The listing builds one solid part. Answer for the finished solid, in the listing's coordinates (mm). Face numbers are marked on the shaded views. A direction names the side the tool comes from. Coordinates: 2 decimals unless noted, no trailing zeros. Loops run counter-clockwise (first coordinate to the right, second up) from the corner with the lowest first, then second, coordinate; pieces in that order, holes last. Notation, with made-up numbers: (54, 20.25) - (81, 20.25) arc R26 ccw to (81, 43.25) - close; hole circle Ø11 at (-38.75, 69). An arc over 180 degrees is marked (long way). Use one line per item in the form item = value. Start each with the question number.
```python
from build123d import *

# Parameters (mm, degrees)
F1_DEPTH = 600
F2_R     = 80
F3_DEPTH = 1200.001
F5_DEPTH = 200.001


with BuildPart() as f1:
    # F0 (on Front) → F1 (new body)
    with BuildSketch(Plane.XZ):
        with BuildLine():
            Line((-800, 100), (-800, -100))
            Line((-800, -100), (800, -100))
            Line((800, -100), (800, 100))
            Line((800, 100), (400, 100))
            Line((400, 100), (400, 500))
            Line((400, 500), (300, 500))
            ThreePointArc((300, 500), (0, 200), (-300, 500))
            Line((-300, 500), (-400, 500))
            Line((-400, 500), (-400, 100))
            Line((-400, 100), (-800, 100))
        make_face()
    extrude(amount=F1_DEPTH)

    # F2 (on face) → F3 (cut, through all)
    with BuildSketch(Plane(origin=(-400, 0, 0), x_dir=(0, -1, 0), z_dir=(-1, 0, 0))):
        with Locations((300, 350)):
            Circle(F2_R)
    extrude(amount=-F3_DEPTH, mode=Mode.SUBTRACT)

    # F4 (on face) → F5 (cut, through all)
    with BuildSketch(Plane.XY.offset(100)):
        with BuildLine():
            ThreePointArc((590, -450), (650, -510), (710, -450))
            Line((710, -450), (710, -150))
            ThreePointArc((710, -150), (650, -90), (590, -150))
            Line((590, -150), (590, -450))
        make_face()
        with BuildLine():
            Line((-710, -150), (-710, -450))
            ThreePointArc((-710, -450), (-650, -510), (-590, -450))
            Line((-590, -450), (-590, -150))
            ThreePointArc((-590, -150), (-650, -90), (-710, -150))
        make_face()
    extrude(amount=-F5_DEPTH, mode=Mode.SUBTRACT)


solid = f1.part
```
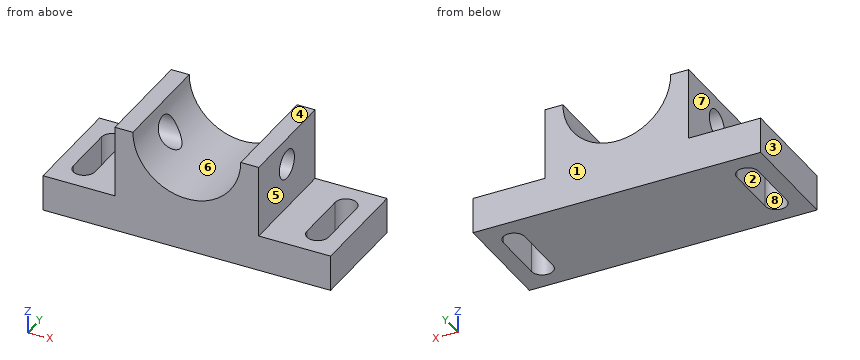
(1) Find the intervals of material crossed by probe 1 along X at (y, z) = (-439, -59); probe 2 along Y at (x, z) = (-340, 350); probe 3 along Z at (x, y) = (317, -300), in increasing order. Write a range as from..to.
(2) A cutting plane is placed at A-A (y = -187.5). Determine the outline of the cut face in (x, z), then the cut area to 3 significant figures.
(3) For the marked faces 4, 5, 6, 7 and 8, determine the directions among +Z, -Z, +X, -X, +Y, -Y from which every point of the face is accessible in a straight line to the end or side of a thin tool.
(4) A cutting plane is placed at D-D (z = 5.5). Determine the outline of the cut face in (x, y), then the cut area to 3 significant figures.
(5) Each of these flat-tipped pins is pushed along its axis until it touches: pin 1 Ø5 at (x, y) = (575.5, -295.5) entering from +Z; pin 2 Ø2 at (y, z) = (-464.5, 359.5) entering from -X; pin 3 Ø6 at (x, y) = (176, -213.5) entering from +Z. Where does it stop, or does it pass through?
(6) Determine the mould class of the marked faces 1, 2 and 3 for opening direction X: +X half, -X half, draft (parallel to the pull), parting line (faces both ways), or undercut.
(7) A cutting plane is placed at B-B (x = 650). Determine the outline of the cut face in (y, z).
(8) A cutting plane is placed at C-C (z = 350). Determine the outline of the cut face in (x, y).
Evaluation:
q1.probe_1 = -800..-710, -590..590, 710..800
q1.probe_2 = -600..-380, -220..0
q1.probe_3 = -100..270, 430..500
q2.outline = (-800, -100) - (-710, -100) - (-710, 100) - (-800, 100) - close; (-590, -100) - (590, -100) - (590, 100) - (400, 100) - (400, 500) - (300, 500) arc R300 cw to (-300, 500) - (-400, 500) - (-400, 100) - (-590, 100) - close; (710, -100) - (800, -100) - (800, 100) - (710, 100) - close
q2.area = 451,000 mm^2
q3.face_4 = +Z, +X, -X, +Y, -Y
q3.face_5 = +Z, +X, +Y, -Y
q3.face_6 = +Z, +Y, -Y
q3.face_7 = +Z, -X, +Y, -Y
q3.face_8 = +Z, -Z
q4.outline = (-800, -600) - (800, -600) - (800, 0) - (-800, 0) - close; hole (-710, -450) arc R60 ccw to (-590, -450) - (-590, -150) arc R60 ccw to (-710, -150) - close; hole (590, -450) arc R60 ccw to (710, -450) - (710, -150) arc R60 ccw to (590, -150) - close
q4.area = 865,000 mm^2
q5.pin_1 = 100
q5.pin_2 = -400
q5.pin_3 = 259.25
q6.face_1 = draft
q6.face_2 = undercut
q6.face_3 = -X half
q7.outline = (-600, -100) - (-510, -100) - (-510, 100) - (-600, 100) - close; (-90, -100) - (0, -100) - (0, 100) - (-90, 100) - close
q8.outline = (-400, -600) - (-259.81, -600) - (-259.81, -380) - (-400, -380) - close; (-400, -220) - (-259.81, -220) - (-259.81, 0) - (-400, 0) - close; (259.81, -600) - (400, -600) - (400, -380) - (259.81, -380) - close; (259.81, -220) - (400, -220) - (400, 0) - (259.81, 0) - close
